```python
from build123d import *

# Parameters (mm, degrees)
SKETCH1_W           = 11.699975178
SKETCH1_H           = 11.699996949
SKETCH1_W_2         = 11.699990436
SKETCH1_H_2         = 11.699981689
SKETCH1_W_3         = 11.699990437
SKETCH1_H_3         = 11.699975177
SKETCH1_W_4         = 11.699981689
SKETCH1_H_4         = 11.699990436
BOSS_EXTRUDE1_DEPTH = 1828.8


with BuildPart() as part:
    # Sketch1 → Boss-Extrude1 (new body)
    with BuildSketch(Plane.XY):
        Polygon((22.500515052, 22.499297556), (-22.499484399, 22.499298105), (-22.499484948, -22.500701346), (-4.249491942, -22.500701568), (-4.249491942, -22.200733242), (-4.24949208, -18.000719999), (-6.799479919, -18.000719999), (-6.799480207, -9.200732353), (-4.799480391, -7.200732362), (4.800525817, -7.200732047), (6.8005258, -9.200731855), (6.800526088, -18.000720263), (4.250507877, -18.000720263), (4.250508015, -22.200733153), (4.250508015, -22.500701672), (22.500514502, -22.500701895), (22.500514725, -4.250714302), (22.200520351, -4.250714302), (18.000507108, -4.25071444), (18.000507108, -6.800702279), (9.200519462, -6.800702567), (7.200519471, -4.800702751), (7.200519156, 4.799303458), (9.200518964, 6.79930344), (18.000507424, 6.799303729), (18.000507424, 4.249285514), (22.200520261, 4.249285652), (22.500514829, 4.249285652), align=None)
        with BuildLine():
            Line((-4.249491247, 17.999291576), (-4.249490956, 22.199304807))
            Line((-4.249490956, 22.199304807), (-3.949472548, 22.199304807))
            Line((-3.949472548, 22.199304807), (-3.481695222, 21.73152644))
            ThreePointArc((-3.481695222, 21.73152644), (-2.670636178, 21.189593132), (-1.713926324, 20.999291428))
            Line((-1.713926324, 20.999291428), (1.714975167, 20.999291428))
            ThreePointArc((1.714975167, 20.999291428), (2.671722509, 21.189608628), (3.482801459, 21.731583767))
            Line((3.482801459, 21.731583767), (3.950490798, 22.199304487))
            Line((3.950490798, 22.199304487), (4.250509108, 22.199304487))
            Line((4.250509108, 22.199304487), (4.250508817, 17.999291575))
            Line((4.250508817, 17.999291575), (6.800527063, 17.999291575))
            Line((6.800527063, 17.999291575), (6.800526453, 9.199302988))
            Line((6.800526453, 9.199302988), (4.800526064, 7.199302969))
            Line((4.800526064, 7.199302969), (-4.799479817, 7.199303635))
            Line((-4.799479817, 7.199303635), (-6.799479854, 9.199304042))
            Line((-6.799479854, 9.199304042), (-6.799479244, 17.999291576))
            Line((-6.799479244, 17.999291576), (-4.249491247, 17.999291576))
        make_face(mode=Mode.SUBTRACT)
        with BuildLine():
            Line((-22.199510888, 4.249285566), (-17.999497356, 4.249285704))
            Line((-17.999497356, 4.249285704), (-17.999497356, 6.79927354))
            Line((-17.999497356, 6.79927354), (-9.199509947, 6.799273828))
            Line((-9.199509947, 6.799273828), (-7.199509956, 4.799274012))
            Line((-7.199509956, 4.799274012), (-7.199509641, -4.800732197))
            Line((-7.199509641, -4.800732197), (-9.199509449, -6.800732179))
            Line((-9.199509449, -6.800732179), (-17.99949762, -6.800732468))
            Line((-17.99949762, -6.800732468), (-17.99949762, -4.250714253))
            Line((-17.99949762, -4.250714253), (-22.199510799, -4.250714391))
            Line((-22.199510799, -4.250714391), (-22.199510799, -3.950696126))
            Line((-22.199510799, -3.950696126), (-21.731790056, -3.48300681))
            ThreePointArc((-21.731790056, -3.48300681), (-21.189814855, -2.671927844), (-20.999497617, -1.71518046))
            Line((-20.999497617, -1.71518046), (-20.999497617, 1.713721031))
            ThreePointArc((-20.999497617, 1.713721031), (-21.189799286, 2.670430863), (-21.731732544, 3.481489907))
            Line((-21.731732544, 3.481489907), (-22.199510888, 3.949267256))
            Line((-22.199510888, 3.949267256), (-22.199510888, 4.249285566))
        make_face(mode=Mode.SUBTRACT)
        with Locations((-14.649542346, -14.650709384)):
            Rectangle(SKETCH1_W, SKETCH1_H, mode=Mode.SUBTRACT)
        with Locations((14.65050626, -14.650767962)):
            Rectangle(SKETCH1_W_2, SKETCH1_H_2, mode=Mode.SUBTRACT)
        with BuildLine():
            Line((-3.181457266, -4.596908447), (-4.595670829, -3.182694885))
            Line((-4.595670829, -3.182694885), (-3.26221457, -1.849238626))
            ThreePointArc((-3.26221457, -1.849238626), (-3.749476751, -0.00071437), (-3.26221457, 1.847809887))
            Line((-3.26221457, 1.847809887), (-4.595670829, 3.181266146))
            Line((-4.595670829, 3.181266146), (-3.181457266, 4.595479708))
            Line((-3.181457266, 4.595479708), (-1.848001007, 3.262023449))
            ThreePointArc((-1.848001007, 3.262023449), (0.000523249, 3.74928563), (1.849047505, 3.262023449))
            Line((1.849047505, 3.262023449), (3.182503764, 4.595479708))
            Line((3.182503764, 4.595479708), (4.596717327, 3.181266146))
            Line((4.596717327, 3.181266146), (3.263261068, 1.847809887))
            ThreePointArc((3.263261068, 1.847809887), (3.750523249, -0.00071437), (3.263261068, -1.849238626))
            Line((3.263261068, -1.849238626), (4.596717327, -3.182694885))
            Line((4.596717327, -3.182694885), (3.182503764, -4.596908447))
            Line((3.182503764, -4.596908447), (1.849047505, -3.263452188))
            ThreePointArc((1.849047505, -3.263452188), (0.000523249, -3.75071437), (-1.848001007, -3.263452188))
            Line((-1.848001007, -3.263452188), (-3.181457266, -4.596908447))
        make_face(mode=Mode.SUBTRACT)
        with Locations((-14.64949028, 14.649335967)):
            Rectangle(SKETCH1_W_3, SKETCH1_H_3, mode=Mode.SUBTRACT)
        with Locations((14.650561583, 14.6492839)):
            Rectangle(SKETCH1_W_4, SKETCH1_H_4, mode=Mode.SUBTRACT)
    extrude(amount=BOSS_EXTRUDE1_DEPTH)


solid = part.part
```
Model file for the job. Use its own axes, mm. Give positions to 0.01 mm unless a question says otherwise; leave off trailing zeros. Use one line per item in the form item = value.
Item 1: Flat gauge pin, fed straight in: pin 1 Ø3 at (y, z) = (-1.5, 1046) entering from +X. Where does the tip first touch, or does it go through?
Filled in:
pin_1 = 7.2
Item 2: Slice it at A-A on z = 1680.5. Give the number of separate pieces and of enclosed holes in the cut face, and give its area (3 significant figures).
Filled in:
separate_pieces = 1
enclosed_holes = 7
area = 715 mm^2
Item 3: Drill centre lines: L1, parallel to X at y = 9, z = 706.5; L2, parallel to X at y = -18.5, z = 562; L3, parallel to X at y = -2.5, z = 1507. Where is each one in solid material? Low to high.
Filled in:
L1 = -22.5 to -20.5, -8.8 to -6.6, 6.6 to 8.8, 20.5 to 22.5
L2 = -22.5 to -20.5, -8.8 to -4.25, 4.25 to 8.8, 20.5 to 22.5
L3 = -22.5 to -21.13, -7.2 to -3.91, 3.91 to 7.2
